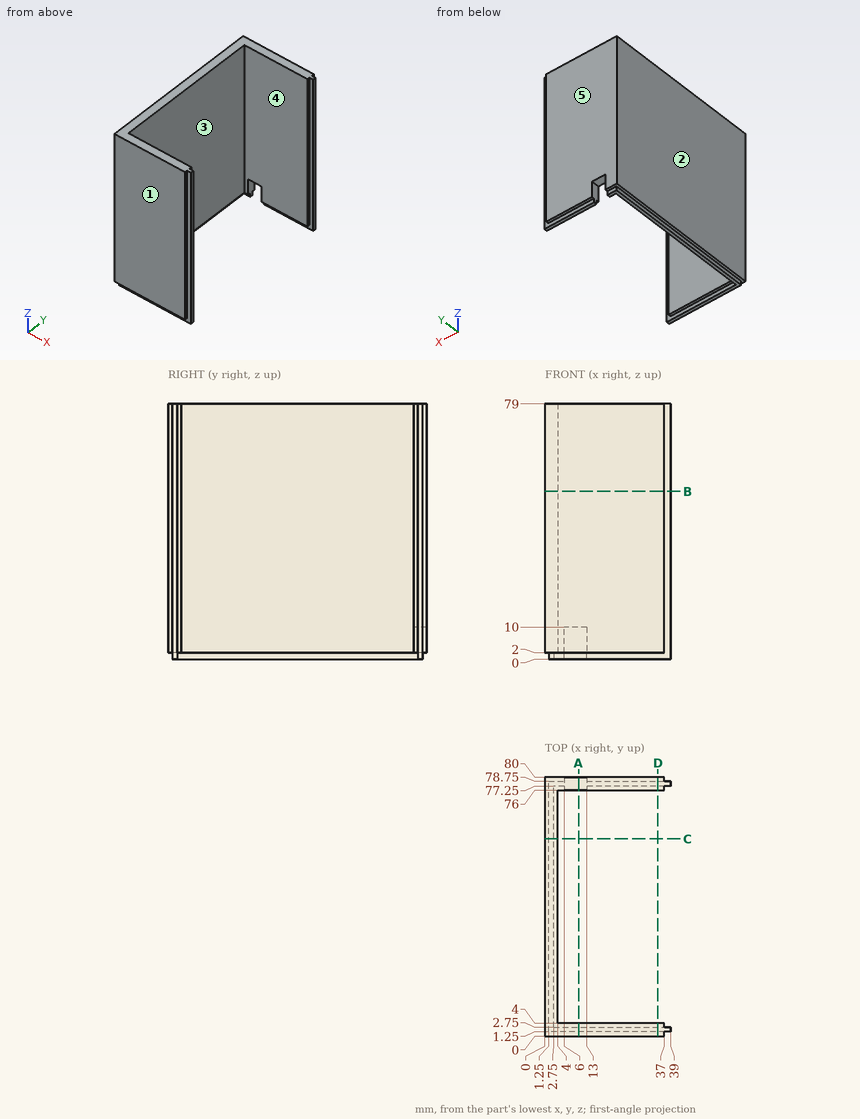
Here's the drawing with two shaded views (mm, measured from the low corner). I have some questions. A direction names the side the tool comes from. Round coordinates to 2 decimals unless told otherwise and drop trailing zeros. Order: outer loops, then holes, each group sorted by start corner. A loop starts at its lowest first (then second) coordinate and runs counter-clockwise, first axis right, second up. Notation, with made-up numbers: M 2,83 L 17,83 A21 ccw 17,94 Z; hole C -4.5,63 d3. An arc over 180 degrees is marked long. Answer in a Markdown table with one row per item.
Item 1: If I drill on L1, parallel to Y at x = 19.5, z = 10; L2, parallel to X at y = 52.5, z = 63; L3, parallel to Z at x = 3.5, y = 20.5, over which ranges is the centre line in solid material (lowest first)? Write a range as from..to.
A:
| item | result |
|---|---|
| L1 | y = 0..4, 76..80 |
| L2 | x = 0..4 |
| L3 | z = 2..79 |
Item 2: Imagine slicing it at C-C, the plane y = 61. Write out the boundary of the cut face in (x, z).
A:
| item | result |
|---|---|
| outline | M 0,2 L 1.25,2 L 1.25,0 L 2.75,0 L 2.75,2 L 4,2 L 4,79 L 0,79 Z |
Item 3: Imagine slicing it at B-B, the plane z = 52. Write out the boundary of the cut face in (x, y), and give its area (3 significant figures).
A:
| item | result |
|---|---|
| outline | M 0,0 L 37,0 L 37,1.25 L 39,1.25 L 39,2.75 L 37,2.75 L 37,4 L 4,4 L 4,76 L 37,76 L 37,77.25 L 39,77.25 L 39,78.75 L 37,78.75 L 37,80 L 0,80 Z |
| area | 590 mm2 |
Item 4: Imagine slicing it at A-A, the plane x = 10.5. Write out the boundary of the cut face in (y, z).
A:
| item | result |
|---|---|
| outline | M 0,2 L 1.25,2 L 1.25,0 L 2.75,0 L 2.75,2 L 4,2 L 4,79 L 0,79 Z; M 76,10 L 80,10 L 80,79 L 76,79 Z |
Item 5: I'm going to push flat-ended pins straight in: pin 1 (5 mm diameter, centred on y = 47, z = 69.5, fed in from +X); pin 2 (1.2 mm diameter, centred on x = 9.5, y = 78.5, fed in from -Z); pin 3 (1.4 mm diameter, centred on y = 0.5, z = 47.5, fed in from +X). Where does each tip first touch, or does it pass through?
A:
| item | result |
|---|---|
| pin 1 | stops at x = 4 |
| pin 2 | stops at z = 10 |
| pin 3 | stops at x = 37 |
Item 6: Thinking about a two-plate mould opening in Y: for the marked faces 1, 2 and 3, which applies, +Y half, -Y half, draft (parallel to the pull), parting line (faces both ways), or undercut?
A:
| item | result |
|---|---|
| face 1 | -Y half |
| face 2 | draft |
| face 3 | undercut |
Item 7: For the marked faces 4 and 5, which set-ups out of +Z, -Z, +X, -X, +Y, -Y let a thin tool reach every point of the face, with its end or its side?
A:
| item | result |
|---|---|
| face 4 | +Z, -Z, +X |
| face 5 | +Z, -Z, +X, -X, +Y |
Item 8: Imagine slicing it at D-D, the plane x = 35. Write out the boundary of the cut face in (y, z), and give its area (3 significant figures).
A:
| item | result |
|---|---|
| outline | M 0,2 L 1.25,2 L 1.25,0 L 2.75,0 L 2.75,2 L 4,2 L 4,79 L 0,79 Z; M 76,2 L 77.25,2 L 77.25,0 L 78.75,0 L 78.75,2 L 80,2 L 80,79 L 76,79 Z |
| area | 622 mm2 |
